```python
from build123d import *


with BuildPart() as part:
    # Sketch1 → Revolve1 (revolve)
    with BuildSketch(Plane.XY, mode=Mode.PRIVATE) as revolve1_sk:
        with BuildLine():
            Line((0, 3.302), (15.24, 3.302))
            Line((15.24, 3.302), (15.24, 9.525))
            Line((15.24, 9.525), (13.810625, 9.525))
            ThreePointArc((13.810625, 9.525), (12.62, 8.334375), (11.429375, 9.525))
            Line((11.429375, 9.525), (10, 9.525))
            Line((10, 9.525), (10, 7.302))
            Line((10, 7.302), (2, 7.302))
            Line((2, 7.302), (2, 9.525))
            Line((2, 9.525), (0, 9.525))
            Line((0, 9.525), (0, 3.302))
        make_face()
    revolve(revolve1_sk.sketch.rotate(Axis((0, 0, 0), (1, 0, 0)), 90), axis=Axis((0, 0, 0), (1, 0, 0)))


solid = part.part
```
For this review, take the finished solid that the model builds, in its own axes (mm). A direction names the side the tool comes from. Round coordinates to 2 decimals unless told otherwise and drop trailing zeros. Order: outer loops, then holes, each group sorted by start corner. A loop starts at its lowest first (then second) coordinate and runs counter-clockwise, first axis right, second up.
Q1. Mouldability with a two-part tool opening along Y and no side actions: class faces 1 (the flat face through (15.24, 0, -4)), 2 (the cylindrical face through (10.7, 9.3, -2.06)), 3 (the cylindrical face through (7.73, -0.99, 3.15)) as pulls with the +Y half, pulls with the -Y half, needs draft (parallel to the pull), parting line crosses it, or undercut.
Findings below:
face 1: needs draft
face 2: parting line crosses it
face 3: undercut
Q2. Insertion check: P1, Ø1.5, axis at x = 8.5, y = 0.5, coming from the +Z side; P2, Ø1, axis at x = 7, y = 1, coming from the -Z side; P3, Ø1.5, axis at x = 8.5, z = 3.5, coming from the -Y side; P4, Ø6, axis at y = 0, z = 0, coming from the -X side. Each pin has a flat end and moves straight along its axis. Give the tip position at first contact, or say it passes through.
Findings below:
P1: stops at z = 7.3
P2: stops at z = -7.28
P3: stops at y = -6.76
P4: passes through
Q3. We need section C-C, the plane x = 6. Give the boundary of the cut face in (y, z).
Findings below:
outline: circle Ø14.6 at (0, 0); hole circle Ø6.6 at (0, 0)
Q4. We need section A-A, the plane z = 0. Give the boundary of the cut face in (x, y) (3 decimals), plus the area to 3 significant figures.
Findings below:
outline: (0, -9.525) - (2, -9.525) - (2, -7.302) - (10, -7.302) - (10, -9.525) - (11.429, -9.525) arc R1.191 cw to (13.811, -9.525) - (15.24, -9.525) - (15.24, -3.302) - (0, -3.302) - close; (0, 3.302) - (15.24, 3.302) - (15.24, 9.525) - (13.811, 9.525) arc R1.191 cw to (11.429, 9.525) - (10, 9.525) - (10, 7.302) - (2, 7.302) - (2, 9.525) - (0, 9.525) - close
area: 150 mm2
Q5. Machinability: for faces 4 (the flat face through (2, 6, -5)), 5 (the flat face through (0, 0, 4)), which of the approach directions +Z, -Z, +X, -X, +Y, -Y give a long, thin tool a straight path to every point of the face, cutting with its end or side? Answer none if there is none.
Findings below:
face 4: none
face 5: +Z, -Z, -X, +Y, -Y
Q6. Wall thickness on line 1 (Y direction, x = 4.5, z = 0); line 2 (X direction, y = 7.75, z = 0.5); line 3 (X direction, y = 7.75, z = -4.25): over which ranges is each line inside the solid? List them lowest first.
Findings below:
line 1: y = -7.3 to -3.3, 3.3 to 7.3
line 2: x = 0 to 2, 10 to 15.24
line 3: x = 0 to 2, 10 to 11.65, 13.59 to 15.24
